from build123d import *

# Parameters (mm, degrees)
SKETCH1_R                  = 1
BASE_SHAPE_DEPTH           = 1
FILLETS_R                  = 1
M2_COUNTERSUNKS_AT_2_COUNT = 2
M2_COUNTERSUNKS_AT_2_PITCH = 73.76
M2_COUNTERSUNKS_AT_3_COUNT = 2
M2_COUNTERSUNKS_AT_3_PITCH = 73.537756289
M2_COUNTERSUNKS_AT_4_COUNT = 2
M2_COUNTERSUNKS_AT_4_PITCH = 92.959345953
M2_COUNTERSUNKS_AT_5_COUNT = 2
M2_COUNTERSUNKS_AT_5_PITCH = 36.88


with BuildPart() as part:
    # Sketch1 → Base shape (new body)
    with BuildSketch(Plane(origin=(0, 0, 0), x_dir=(1, 0, 0), z_dir=(0, 1, 0))):
        with BuildLine():
            ThreePointArc((2.75, 36.88), (1.944543648, 34.935456352), (0, 34.13))
            Line((0, 34.13), (-63.992025159, 34.13))
            ThreePointArc((-63.992025159, 34.13), (-70.681255309, 31.35923015), (-73.452025159, 24.67))
            ThreePointArc((-73.452025159, 24.67), (-71.507481511, 23.864543648), (-70.702025159, 21.92))
            ThreePointArc((-70.702025159, 21.92), (-71.507481511, 19.975456352), (-73.452025159, 19.17))
            Line((-73.452025159, 19.17), (-73.452025159, 16.662625843))
            ThreePointArc((-73.452025159, 16.662625843), (-63.663567803, 10.763596053), (-59.822025159, 0))
            ThreePointArc((-59.822025159, 0), (-63.663567803, -10.763596053), (-73.452025159, -16.662625843))
            Line((-73.452025159, -16.662625843), (-73.452025159, -19.17))
            ThreePointArc((-73.452025159, -19.17), (-71.507481511, -19.975456352), (-70.702025159, -21.92))
            ThreePointArc((-70.702025159, -21.92), (-71.507481511, -23.864543648), (-73.452025159, -24.67))
            Line((-73.452025159, -24.67), (-73.452025159, -30.8))
            Line((-73.452025159, -30.8), (-63.952025159, -30.8))
            Line((-63.952025159, -30.8), (-63.952025159, -34.13))
            Line((-63.952025159, -34.13), (-63.952025159, -39.5))
            Line((-63.952025159, -39.5), (-53.952025159, -39.5))
            Line((-53.952025159, -39.5), (-48.582025159, -34.13))
            Line((-48.582025159, -34.13), (0, -34.13))
            ThreePointArc((0, -34.13), (1.944543648, -34.935456352), (2.75, -36.88))
            ThreePointArc((2.75, -36.88), (2.220381771, -38.502468734), (0.835523788, -39.5))
            Line((0.835523788, -39.5), (11.4, -39.5))
            Line((11.4, -39.5), (11.4, 39.5))
            Line((11.4, 39.5), (0.835523788, 39.5))
            ThreePointArc((0.835523788, 39.5), (2.220381771, 38.502468734), (2.75, 36.88))
        make_face()
        with Locations(Location((-64.925, -21.92, 0), (0, 0, 270))):
            Circle(SKETCH1_R, mode=Mode.SUBTRACT)
        with Locations(Location((7.075, -36.88, 0), (0, 0, 270))):
            Circle(SKETCH1_R, mode=Mode.SUBTRACT)
        with Locations(Location((-64.925, 21.92, 0), (0, 0, 270))):
            Circle(SKETCH1_R, mode=Mode.SUBTRACT)
        with Locations(Location((7.075, 0, 0), (0, 0, 270))):
            Circle(SKETCH1_R, mode=Mode.SUBTRACT)
        with Locations(Location((7.075, 36.88, 0), (0, 0, 270))):
            Circle(SKETCH1_R, mode=Mode.SUBTRACT)
    extrude(amount=BASE_SHAPE_DEPTH)

    # Fillets
    fillets_edges = [part.edges().sort_by_distance(p)[0] for p in [
        (0.835523788, 0.5, -39.5),
        (11.4, 0.5, -39.5),
        (11.4, 0.5, 39.5),
        (0.835523788, 0.5, 39.5),
        (-48.582025159, 0.5, 34.13),
        (-53.952025159, 0.5, 39.5),
        (-63.952025159, 0.5, 30.8),
        (-73.452025159, 0.5, 30.8),
        (-73.452025159, 0.5, 24.67),
        (-73.452025159, 0.5, 19.17),
        (-73.452025159, 0.5, 16.662625843),
        (-73.452025159, 0.5, -16.662625843),
        (-73.452025159, 0.5, -19.17),
        (-73.452025159, 0.5, -24.67),
    ]]
    fillet(fillets_edges, radius=FILLETS_R)

    # Sketch3 → M2 countersunks (revolve, cut)
    with BuildSketch(Plane(origin=(7.075, 0, -36.88), x_dir=(0, 0, -1), z_dir=(1, 0, 0))):
        Polygon((0, 0), (0, 1), (1, 1), (1, 1.1), (2, 0.1), (2, 0), align=None)
    m2_countersunks = revolve(axis=Axis((7.075, -6.35, -36.88), (0, 1, 0)), mode=Mode.SUBTRACT)

    # M2 countersunks at 2: M2 countersunks ×2
    with Locations(*[(0, 0, i * M2_COUNTERSUNKS_AT_2_PITCH) for i in range(1, M2_COUNTERSUNKS_AT_2_COUNT)]):
        add(m2_countersunks, mode=Mode.SUBTRACT)

    # M2 countersunks at 3: M2 countersunks ×2
    with Locations(*[Vector(-0.9790888875801275, 0, 0.2034329133083154) * (i * M2_COUNTERSUNKS_AT_3_PITCH) for i in range(1, M2_COUNTERSUNKS_AT_3_COUNT)]):
        add(m2_countersunks, mode=Mode.SUBTRACT)

    # M2 countersunks at 4: M2 countersunks ×2
    with Locations(*[Vector(-0.7745321275866415, 0, 0.6325345708624239) * (i * M2_COUNTERSUNKS_AT_4_PITCH) for i in range(1, M2_COUNTERSUNKS_AT_4_COUNT)]):
        add(m2_countersunks, mode=Mode.SUBTRACT)

    # M2 countersunks at 5: M2 countersunks ×2
    with Locations(*[(0, 0, i * M2_COUNTERSUNKS_AT_5_PITCH) for i in range(1, M2_COUNTERSUNKS_AT_5_COUNT)]):
        add(m2_countersunks, mode=Mode.SUBTRACT)


solid = part.part
Geometry: final body of the model. Coordinates: model frame, mm. Give positions to 0.01 mm unless a question says otherwise; leave off trailing zeros. Order: outer loops, then holes, each group sorted by start corner. A loop starts at its lowest first (then second) coordinate and runs counter-clockwise, first axis right, second up. Notation, with made-up numbers: (11, 69) -> (58, 69) arc R16 ccw to (58, 79) -> close; hole circle Ø5 at (38, 1.25). An arc over 180 degrees is marked (long way). Answer as a JSON object with one key per item and string values.
Q1. First-contact query: pin 1 (6.5 mm diameter, centred on x = 7.075, z = 0, fed in from -Y); pin 2 (3.5 mm diameter, centred on x = -64.925, z = 21.92, fed in from -Y). Flat tips, straight axial feed; report the tip coordinate or a pass-through.
Entries:
{"pin 1": "stops at y = 0", "pin 2": "stops at y = 0.35"}
Q2. Draft query along X for faces 1 (the flat face through (-32, 1, -1)), 2 (the cylindrical face through (-70.263, 0.493, -31.753)), 3 (the flat face through (-51.3, 0.49, 36.85)). Return one class per face: released by +X, released by -X, zero draft, split by the parting line, or undercut.
Entries:
{"face 1": "zero draft", "face 2": "released by -X", "face 3": "undercut"}
Q3. Material intervals for probe 1 along X at (y, z) = (0.1, -36.88) (3 decimals); probe 2 along X at (y, z) = (0.05, 21.92) (3 decimals); probe 3 along Z at (x, y) = (-16.5, 0.45), sorted ascending.
Entries:
{"probe 1": "x = 2.75 to 5.075, 9.075 to 11.4", "probe 2": "x = -70.702 to -66.925, -62.925 to 11.4", "probe 3": "z = -34.13 to 34.13"}
Q4. Section A-A (y = 0.3). State how many separate pieces and enclosed holes the cut face has, plus the area to 3 significant figures.
Entries:
{"separate pieces": "1", "enclosed holes": "5", "area": "5,490 mm^2"}
Q5. Section B-B (x = -30). Output: boundary loops of the cut face in (y, z), plus the area to 3 significant figures.
Entries:
{"outline": "(0, -34.13) -> (1, -34.13) -> (1, 34.13) -> (0, 34.13) -> close", "area": "68.3 mm^2"}
